Check sheet for the modelled part. Datum: model origin and axes. Units: mm. A direction names the side the tool comes from. Round coordinates to 2 decimals unless told otherwise and drop trailing zeros. Loops run counter-clockwise (first coordinate to the right, second up) from the corner with the lowest first, then second, coordinate; pieces in that order, holes last. Notation, with made-up numbers: (-1.5, 41.5) - (35.5, 41.5) arc R20 cw to (35.5, 71.5) - close; hole circle Ø8 at (24, 28). An arc over 180 degrees is marked (long way). Return JSON: item names as keys, results as strings.
from build123d import *

# Parameters (mm, degrees)
BOSS_EXTRUDE1_DEPTH          = 25.4
F_1_1_0000_DOWEL_HOLE1_D     = 25.4
F_1_1_0000_DOWEL_HOLE1_DEPTH = 6.35
F_1_1_0000_DOWEL_HOLE1_TIP   = 7.630929862


with BuildPart() as part:
    # Sketch2 → Boss-Extrude1 (new body)
    with BuildSketch(Plane(origin=(0, 0, 0), x_dir=(0, 0, -1), z_dir=(1, 0, 0))):
        with BuildLine():
            Line((-25.20103811, 26.834337713), (20.51896189, 26.834337713))
            ThreePointArc((20.51896189, 26.834337713), (22.315013114, 26.090388938), (23.05896189, 24.294337713))
            Line((23.05896189, 24.294337713), (23.05896189, -21.425662287))
            ThreePointArc((23.05896189, -21.425662287), (22.315013114, -23.221713511), (20.51896189, -23.965662287))
            Line((20.51896189, -23.965662287), (-25.20103811, -23.965662287))
            ThreePointArc((-25.20103811, -23.965662287), (-26.997089334, -23.221713511), (-27.74103811, -21.425662287))
            Line((-27.74103811, -21.425662287), (-27.74103811, 24.294337713))
            ThreePointArc((-27.74103811, 24.294337713), (-26.997089334, 26.090388938), (-25.20103811, 26.834337713))
        make_face()
    extrude(amount=BOSS_EXTRUDE1_DEPTH)

    # 1 (1.0000) Dowel Hole1
    with Locations(Plane(origin=(25.4, 0, 0), x_dir=(0, 0, -1), z_dir=(1, 0, 0))):
        with Locations((-2.40903604, 2.862294249)):
            Hole(F_1_1_0000_DOWEL_HOLE1_D / 2, depth=F_1_1_0000_DOWEL_HOLE1_DEPTH)
            with Locations((0, 0, -(F_1_1_0000_DOWEL_HOLE1_DEPTH + F_1_1_0000_DOWEL_HOLE1_TIP / 2))):  # 118° drill point
                Cone(0, F_1_1_0000_DOWEL_HOLE1_D / 2, F_1_1_0000_DOWEL_HOLE1_TIP, mode=Mode.SUBTRACT)


solid = part.part
Q1. Sectioned sample at A-A (x = 20). Enter the section's corners in (y, z).
Answer key:
{"outline": "(-23.97, -20.52) arc R2.54 ccw to (-21.43, -23.06) - (24.29, -23.06) arc R2.54 ccw to (26.83, -20.52) - (26.83, 25.2) arc R2.54 ccw to (24.29, 27.74) - (-21.43, 27.74) arc R2.54 ccw to (-23.97, 25.2) - close; hole circle Ø25.4 at (2.86, 2.41)"}
Q2. Tool access check on faces 1 (the face through (12.522, -23.202, -22.335)), 2 (the face through (22.181, -4.865, -7.669)). Record the directions out of +Z, -Z, +X, -X, +Y, -Y that give a thin tool (end or side, any length) a straight path to the whole face; none if there is none.
Answer key:
{"face 1": "-Z, +X, -X, -Y", "face 2": "+X"}
Q3. Sectioned sample at B-B (x = 13.75). Enter the section's corners in (y, z), plus the area to 3 significant figures.
Answer key:
{"outline": "(-23.97, -20.52) arc R2.54 ccw to (-21.43, -23.06) - (24.29, -23.06) arc R2.54 ccw to (26.83, -20.52) - (26.83, 25.2) arc R2.54 ccw to (24.29, 27.74) - (-21.43, 27.74) arc R2.54 ccw to (-23.97, 25.2) - close; hole circle Ø7.76 at (2.86, 2.41)", "area": "2,530 mm²"}
Q4. Depth check by flat-ended pin: P1, Ø2, axis at y = -4.5, z = 8.5, coming from the +X side. Enter the tip coordinate at first touch or a pass-through.
Answer key:
{"P1": "stops at x = 17.76"}
Q5. Draft check along Y on faces 3 (the face through (12.74, 4.35, 4.03)), 4 (the face through (13, 26.834, 3)), 5 (the face through (0, 2, 2)), 6 (the face through (12.52, -23.24, 26.98)). Enter one of: released by +Y, released by -Y, zero draft, split by the parting line, or undercut.
Answer key:
{"face 3": "undercut", "face 4": "released by +Y", "face 5": "zero draft", "face 6": "released by -Y"}
Q6. Scan lines: probe 1 along Z at (x, y) = (20.75, 4.5); probe 2 along Z at (x, y) = (23, -6); probe 3 along Z at (x, y) = (5.25, 25.5). Record each from-to range of solid material in increasing order. Write a range as [from, to].
Answer key:
{"probe 1": "z = [-23.06, -10.18], [15, 27.74]", "probe 2": "z = [-23.06, -6.69], [11.51, 27.74]", "probe 3": "z = [-22.75, 27.44]"}
